Here's how the part is built. I have some questions about the finished solid (model axes, mm). Face numbers are marked on the shaded views. Coordinates: 2 decimals unless noted, no trailing zeros. Write each loop counter-clockwise with the first axis right and the second up, starting at its lowest first coordinate (ties: lowest second). Pieces come first, ordered by that corner, then holes.
Item 1: I want a section at C-C (y = 0.25). Count the separate pieces of the cut face and the enclosed holes in it, and give its area (3 significant figures).
Item 2: I want a section at D-D (z = -3.25). Please give me the cut outline in (x, y).
Item 3: Please list where these lines run through material, in increasing order: line 1 (Z direction, x = -0.75, y = 1.2); line 2 (X direction, y = 0.8, z = -7.25); line 3 (Z direction, x = 5.75, y = 0.55).
Item 4: If we mould it in two halves opening along X, with no side actions, what happens to the marked faces 1, 2, 3 and 4? For each: pulls with the +X half, pulls with the -X half, needs draft (parallel to the pull), parting line crosses it, or undercut.
Item 5: I want a section at B-B (x = 0). Please give me the cut outline in (y, z) (3 decimals), and give its area (3 significant figures).
Item 6: I want a section at A-A (z = 0). Please give me the cut outline in (x, y) (3 decimals).
from build123d import *

# Parameters (mm, degrees)
SKETCH_1_W          = 22.002454374
SKETCH_1_H          = 22.002454374
SKETCH_1_R          = 1.5
EXTRUDE_1_DEPTH     = 2
FILLET_1_R          = 2
SKETCH_3_R          = 1.5
CUT_EXTRUDE_2_DEPTH = 10
SKETCH_4_R          = 5.125
CUT_EXTRUDE_3_DEPTH = 10


with BuildPart() as part:
    # 草图1 → 凸台-拉伸1 (new body)
    with BuildSketch(Plane(origin=(0, 0, 0), x_dir=(1, 0, 0), z_dir=(0, 1, 0))):
        Rectangle(SKETCH_1_W, SKETCH_1_H)
        with Locations(Location((-8.131727984, 8.131727984, 0), (0, 0, 270))):
            Circle(SKETCH_1_R, mode=Mode.SUBTRACT)
        with Locations(Location((8.131727984, -8.131727984, 0), (0, 0, 90))):
            Circle(SKETCH_1_R, mode=Mode.SUBTRACT)
        with Locations(Location((8.131727984, 8.131727984, 0), (0, 0, 270))):
            Circle(SKETCH_1_R, mode=Mode.SUBTRACT)
        with Locations(Location((-8.131727984, -8.131727984, 0), (0, 0, 90))):
            Circle(SKETCH_1_R, mode=Mode.SUBTRACT)
    extrude(amount=EXTRUDE_1_DEPTH)

    # 圆角1
    fillet_1_edges = [part.edges().sort_by_distance(p)[0] for p in [
        (11.001227187, 1, 11.001227187),
        (-11.001227187, 1, 11.001227187),
        (-11.001227187, 1, -11.001227187),
        (11.001227187, 1, -11.001227187),
    ]]
    fillet(fillet_1_edges, radius=FILLET_1_R)

    # 草图3 → 切除-拉伸2 (cut)
    with BuildSketch(Plane(origin=(0, 0, 0), x_dir=(1, 0, 0), z_dir=(0, 1, 0))):
        with Locations(Location((-7, 0, 0), (0, 0, 270))):
            Circle(SKETCH_3_R)
        with Locations(Location((7, 0, 0), (0, 0, 90))):
            Circle(SKETCH_3_R)
        with Locations(Location((0, 7, 0), (0, 0, 270))):
            Circle(SKETCH_3_R)
        with Locations(Location((0, -7, 0), (0, 0, 90))):
            Circle(SKETCH_3_R)
    extrude(amount=CUT_EXTRUDE_2_DEPTH, mode=Mode.SUBTRACT)

    # 草图4 → 切除-拉伸3 (cut)
    with BuildSketch(Plane.XZ):
        with Locations(Location((0, 0, 0), (0, 0, 270))):
            Circle(SKETCH_4_R)
    extrude(amount=-CUT_EXTRUDE_3_DEPTH, mode=Mode.SUBTRACT)


solid = part.part
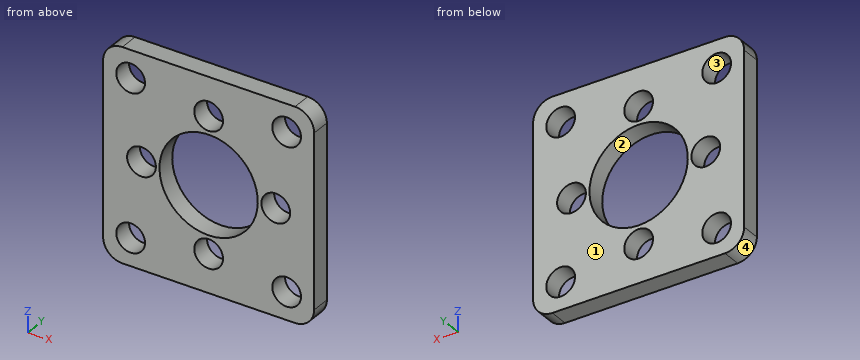
Answer:
1. separate pieces: 1
1. enclosed holes: 9
1. area: 342 mm2
2. outline: (-11, 0) - (-3.96, 0) - (-3.96, 2) - (-11, 2) - close; (3.96, 0) - (11, 0) - (11, 2) - (3.96, 2) - close
3. line 1: z = -11 to -8.3, -5.7 to -5.07, 5.07 to 5.7, 8.3 to 11
3. line 2: x = -11 to -9.35, -6.92 to -1.48, 1.48 to 6.92, 9.35 to 11
3. line 3: z = -11 to -0.83, 0.83 to 11
4. face 1: needs draft
4. face 2: undercut
4. face 3: undercut
4. face 4: pulls with the -X half
5. outline: (0, -11.001) - (2, -11.001) - (2, -8.5) - (0, -8.5) - close; (0, -5.5) - (2, -5.5) - (2, -5.125) - (0, -5.125) - close; (0, 5.125) - (2, 5.125) - (2, 5.5) - (0, 5.5) - close; (0, 8.5) - (2, 8.5) - (2, 11.001) - (0, 11.001) - close
5. area: 11.5 mm2
6. outline: (-11.001, 0) - (-8.5, 0) - (-8.5, 2) - (-11.001, 2) - close; (-5.5, 0) - (-5.125, 0) - (-5.125, 2) - (-5.5, 2) - close; (5.125, 0) - (5.5, 0) - (5.5, 2) - (5.125, 2) - close; (8.5, 0) - (11.001, 0) - (11.001, 2) - (8.5, 2) - close
